Input: part model. Units: mm. Frame: model coordinates. Coordinates: 2 decimals unless noted, no trailing zeros. Loops run counter-clockwise (first coordinate to the right, second up) from the corner with the lowest first, then second, coordinate; pieces in that order, holes last.
Item 1: Section C-C on x = 555. Return loops of the section in (y, z).
Item 2: Ray query, line 1 along Z through (x, y) = (563.5, 263.5); line 2 along X through (y, z) = (231.5, -72); line 3 along Y through (x, z) = (562, -237). Return the intervals inside material, ascending.
Item 3: Contact query for flat-ended pins moving along their axis: P1, Ø1, axis at x = 566.5, y = 288.5, coming from the -Z side; P2, Ø8, axis at x = 563.69, y = 231.72, coming from the +Z side; P3, Ø5, axis at x = 560.5, y = 256, coming from the +Z side; P4, Ø10, axis at x = 568.5, y = 329, coming from the -Z side. Output: stop coordinate, or through.
Item 4: Section A-A on z = -178.5. Return loops of the section in (x, y).
Item 5: Section B-B on y = 272. Return loops of the section in (x, z) (1 decimal), and give its area (3 significant figures).
```python
from build123d import *

# Parameters (mm, degrees)
SKETCH1_R           = 12.7
SKETCH1_R_2         = 5
BASE_EXTRUDE_DEPTH  = 12.7
SKETCH2_R           = 5
SKETCH2_R_2         = 2.5
BOSS_EXTRUDE1_DEPTH = 282.575
SKETCH5_R           = 5.5
SKETCH5_R_2         = 2.5
SKETCH7_R           = 4.7625
SKETCH7_R_2         = 2.5
BOSS_EXTRUDE2_DEPTH = 105.156


with BuildPart() as part:
    # Sketch1 → Base-Extrude (new body)
    with BuildSketch(Plane.XY):
        with Locations((563.692704422, 231.718004299)):
            Circle(SKETCH1_R)
        with Locations((563.692704422, 231.718004299)):
            Circle(SKETCH1_R_2, mode=Mode.SUBTRACT)
    extrude(amount=-BASE_EXTRUDE_DEPTH)

    # Sketch2 → Boss-Extrude1 (add)
    with BuildSketch(Plane.XY):
        with Locations((563.692704422, 231.718004299)):
            Circle(SKETCH2_R)
        with Locations((563.692704422, 231.718004299)):
            Circle(SKETCH2_R_2, mode=Mode.SUBTRACT)
    extrude(amount=-BOSS_EXTRUDE1_DEPTH)

    # Boss-Sweep2: sweep along a path in Sketch6
    with BuildLine(Plane(origin=(563.692704422, 0, 0), x_dir=(0, 0, -1), z_dir=(1, 0, 0))) as boss_sweep2_path:
        ThreePointArc((282.575, 231.718004299), (289.129269744, 234.432871718), (291.844137163, 240.987141462))
    # Sketch5 → Boss-Sweep2 (sweep)
    with BuildSketch(Plane(origin=(0, 0, -282.575), x_dir=(-1, 0, 0), z_dir=(0, 0, -1))):
        with Locations((-563.692704422, 231.718004299)):
            Circle(SKETCH5_R)
        with Locations((-563.692704422, 231.718004299)):
            Circle(SKETCH5_R_2, mode=Mode.SUBTRACT)
    sweep(path=boss_sweep2_path.line)

    # Sketch7 → Boss-Extrude2 (add)
    with BuildSketch(Plane(origin=(0, 240.987141462, 0), x_dir=(-1, 0, 0), z_dir=(0, 1, 0))):
        with Locations(Location((-563.692704422, -291.844137163, 0), (0, 0, 90))):
            Circle(SKETCH7_R)
        with Locations(Location((-563.692704422, -291.844137163, 0), (0, 0, 270))):
            Circle(SKETCH7_R_2, mode=Mode.SUBTRACT)
    extrude(amount=BOSS_EXTRUDE2_DEPTH)


solid = part.part
```
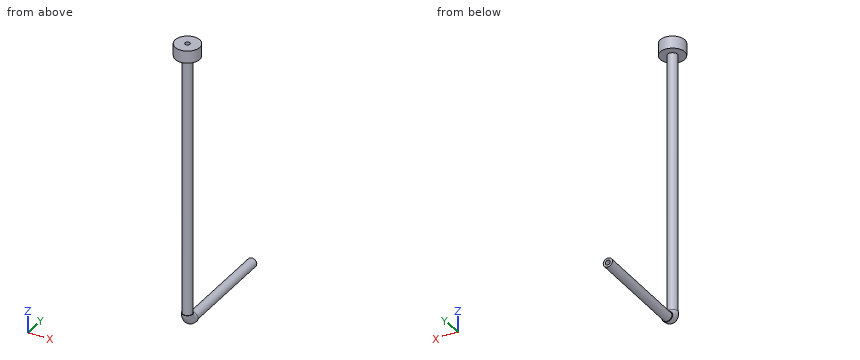
Results found:
1. outline: (222.46, -12.7) - (240.98, -12.7) - (240.98, 0) - (222.46, 0) - close
2. line 1: z = -296.6 to -294.34, -289.35 to -287.09
2. line 2: x = 558.7 to 561.2, 566.18 to 568.69
2. line 3: y = 227.01 to 229.88, 233.56 to 236.42
3. P1: stops at z = -296.01
3. P2: stops at z = 0
3. P3: stops at z = -287.13
3. P4: stops at z = -296.61
4. outline: circle Ø10 at (563.69, 231.72); hole circle Ø5 at (563.69, 231.72)
5. outline: circle Ø9.5 at (563.7, -291.8); hole circle Ø5 at (563.7, -291.8)
5. area: 51.6 mm2
